```python
from build123d import *

# Parameters (mm, degrees)
SKETCH1_R           = 4.75
BOSS_EXTRUDE1_DEPTH = 7
SKETCH2_R           = 2.5
BOSS_EXTRUDE2_DEPTH = 6
SKETCH3_R           = 5
SKETCH3_R_2         = 2.5
BOSS_EXTRUDE3_DEPTH = 3
SKETCH4_R           = 4
SKETCH4_R_2         = 2.5
BOSS_EXTRUDE4_DEPTH = 1.5
FILLET2_R           = 1
FILLET3_R           = 1
SKETCH5_R           = 5.5
SKETCH5_R_2         = 2.5
BOSS_EXTRUDE5_DEPTH = 1.5


with BuildPart() as part:
    # Sketch1 → Boss-Extrude1 (new body)
    with BuildSketch(Plane.XY):
        Circle(SKETCH1_R)
        Polygon((0, 1.5), (-1.299038106, 0.75), (-1.299038106, -0.75), (0, -1.5), (1.299038106, -0.75), (1.299038106, 0.75), align=None, mode=Mode.SUBTRACT)
    extrude(amount=BOSS_EXTRUDE1_DEPTH)

    # Sketch2 → Boss-Extrude2 (add)
    with BuildSketch(Plane.XY.offset(7)):
        Polygon((0, 5.75), (-4.979646072, 2.875), (-4.979646072, -2.875), (0, -5.75), (4.979646072, -2.875), (4.979646072, 2.875), align=None)
        Circle(SKETCH2_R, mode=Mode.SUBTRACT)
    extrude(amount=BOSS_EXTRUDE2_DEPTH)

    # Sketch3 → Boss-Extrude3 (add)
    with BuildSketch(Plane.XY.offset(13)):
        with Locations(Location((0, 0, 0), (0, 0, 174.828408841))):
            Circle(SKETCH3_R)
        Circle(SKETCH3_R_2, mode=Mode.SUBTRACT)
    extrude(amount=BOSS_EXTRUDE3_DEPTH)

    # Sketch4 → Boss-Extrude4 (add)
    with BuildSketch(Plane.XY.offset(16)):
        Circle(SKETCH4_R)
        Circle(SKETCH4_R_2, mode=Mode.SUBTRACT)
    extrude(amount=BOSS_EXTRUDE4_DEPTH)

    # Fillet2
    fillet2_edges = [part.edges().sort_by_distance(p)[0] for p in [
        (4.979646072, -0.450693909, 16),
    ]]
    fillet(fillet2_edges, radius=FILLET2_R - 0.0001)  # a hair under: the kernel refuses the full size

    # Fillet3
    fillet3_edges = [part.edges().sort_by_distance(p)[0] for p in [
        (-2.5, 0, 7),
    ]]
    fillet(fillet3_edges, radius=FILLET3_R - 0.0001)  # a hair under: the kernel refuses the full size

    # Sketch5 → Boss-Extrude5 (add)
    with BuildSketch(Plane.XY.offset(17.5)):
        Circle(SKETCH5_R)
        Circle(SKETCH5_R_2, mode=Mode.SUBTRACT)
    extrude(amount=BOSS_EXTRUDE5_DEPTH)


solid = part.part
```
Geometry: final body of the model. Coordinates: model frame, mm. A direction names the side the tool comes from. Round coordinates to 2 decimals unless told otherwise and drop trailing zeros. Order: outer loops, then holes, each group sorted by start corner. A loop starts at its lowest first (then second) coordinate and runs counter-clockwise, first axis right, second up. Notation, with made-up numbers: (76, 4.5) -> (117, 4.5) arc R25 ccw to (117, 16.5) -> close; hole circle Ø9 at (15.5, -21.5). An arc over 180 degrees is marked (long way). Use one line per item in the form item = value.
(1) Section C-C on z = 11.25. Return loops of the section in (x, y) (3 decimals).
Results list:
outline = (-4.98, -2.875) -> (0, -5.75) -> (4.98, -2.875) -> (4.98, 2.875) -> (0, 5.75) -> (-4.98, 2.875) -> close; hole circle Ø5 at (0, 0)
(2) Access query for faces 1 (the face through (-4.48, 2.55, 13)), 2 (the face through (-0.64, 1.13, 3.45)), 3 (the face through (-4, -3, 7)), 4 (the face through (-4, -2, 17.5)), 5 (the face through (-4.4, -2.7, 13)). Directions: +Z, -Z, +X, -X, +Y, -Y. A direction counts if a zero-diameter tool reaches every point of the face in a straight line with its end or side. Return the directions, or none.
Results list:
face_1 = -X, +Y
face_2 = +Z, -Z
face_3 = -Z
face_4 = none
face_5 = -X, -Y
(3) Section B-B on z = 4.75. Return loops of the section in (x, y), and give its area (3 significant figures).
Results list:
outline = circle Ø9.5 at (0, 0); hole (-1.3, -0.75) -> (0, -1.5) -> (1.3, -0.75) -> (1.3, 0.75) -> (0, 1.5) -> (-1.3, 0.75) -> close
area = 65.0 mm^2
(4) First-contact query: pin 1 Ø1.7 at (y, z) = (-0.5, 10) entering from +X; pin 2 Ø0.5 at (x, y) = (-2.5, -4.5) entering from -Z; pin 3 Ø6.5 at (y, z) = (1.5, 9) entering from -X. Flat tips, straight axial feed; report the tip coordinate or a pass-through.
Results list:
pin_1 = 4.98
pin_2 = 7
pin_3 = -4.98
(5) Ray query, probe 1 along Y at (x, z) = (0, 15); probe 2 along Y at (x, z) = (0.25, 8.5); probe 3 along Z at (x, y) = (-4.25, -2.5). Return the intervals inside material, ascending. Write a range as [from, to].
Results list:
probe_1 = [-5, -2.5], [2.5, 5]
probe_2 = [-5.61, -2.49], [2.49, 5.61]
probe_3 = [7, 15.37], [17.5, 19]
(6) Draft query along Y for faces 6 (the face through (0, 5.2, 13)), 7 (the face through (-2.525, -4.292, 9.958)), 8 (the face through (-0.54, -2.44, 13.42)). Return one class per face: pulls with the +Y half, pulls with the -Y half, needs draft (parallel to the pull), parting line crosses it, or undercut.
Results list:
face_6 = needs draft
face_7 = pulls with the -Y half
face_8 = undercut
(7) Section D-D on z = 13.25. Return loops of the section in (x, y).
Results list:
outline = circle Ø10 at (0, 0); hole circle Ø5 at (0, 0)
